Autodesk Inventor part; units mm, degrees
ref_plane "YZ Plane" through (0, 0, 0) normal (1, 0, 0) x (0, 1, 0)
ref_plane "XZ Plane" through (0, 0, 0) normal (0, 1, 0) x (-1, 0, 0)
ref_plane "XY Plane" through (0, 0, 0) normal (0, 0, 1) x (1, 0, 0)
sketch "Sketch1" plane through (0, 0, 0) normal (0, 1, 0) x (-1, 0, 0)
  line L0 (-18.5, 9.5) -> (-18.5, -9.5)
  line L1 (-18.5, -9.5) -> (18.5, -9.5)
  line L2 (18.5, -9.5) -> (18.5, 9.5)
  line L3 (18.5, 9.5) -> (-18.5, 9.5)
  line L4 (-18.5, 9.5) -> (18.5, -9.5) construction
  line L5 (-18.5, -9.5) -> (18.5, 9.5) construction
  point P0 (0, 0)
  dimension "d0" = 19
  dimension "d1" = 37
extrude "Extrusion1" add sketch "Sketch1" along normal blind 1
sketch "Sketch2" plane through (0, 1, 0) normal (0, 1, 0) x (1, 0, 0)
  line L0 (-18.5, 9.5) -> (-18.5, -9.5) construction
  line L1 (18.5, 9.5) -> (-18.5, 9.5) construction
  line L2 (-18.5, -9.5) -> (18.5, 9.5) construction
  line L3 (18.5, -9.5) -> (18.5, 9.5) construction
  line L4 (-18.5, 9.5) -> (18.5, -9.5) construction
  line L5 (-18.5, 0) -> (18.5, 0) construction
  line L6 (0, -9.5) -> (0, 9.5) construction
  line L7 (18.5, 9.5) -> (14.5, 9.5) construction
  line L8 (14.5, 9.5) -> (14.5, 8.5) construction
  line L9 (14.5, 8.5) -> (14.5, 4.5)
  line L10 (14.5, 4.5) -> (4.5, 4.5)
  line L11 (4.5, 4.5) -> (4.5, 8.5)
  line L12 (4.5, 8.5) -> (14.5, 8.5)
  line L13 (4.5, 4.5) -> (14.5, 8.5) construction
  line L14 (4.5, 8.5) -> (14.5, 4.5) construction
  line L15 (6.6893, 4.5) -> (6.6893, 8.5) construction
  line L16 (6.6893, 5.3757) -> (14.5, 5.3757) construction
  line L17 (12.159, 4.5) -> (12.159, 8.5) construction
  line L18 (6.6893, 6.5) -> (12.159, 6.5) construction
  line L19 (6.6893, 8.5) -> (12.159, 8.5)
  line L20 (12.159, 4.5) -> (6.6893, 4.5)
  arc A0 (6.6893, 8.5) -> (6.6893, 4.5) centre (6.6893, 6.5) ccw
  arc A1 (12.159, 4.5) -> (12.159, 8.5) centre (12.159, 6.5) ccw
  line L21 (18.5, 4.5) -> (11.5, 4.5) construction
  line L22 (11.5, 4.5) -> (11.5, 4) construction
  line L23 (11.5, 4) -> (11.5, -2)
  line L24 (11.5, -2) -> (7.5, -2)
  line L25 (7.5, -2) -> (7.5, 4)
  line L26 (7.5, 4) -> (11.5, 4)
  line L27 (7.5, 4) -> (1.5, 4) construction
  line L28 (1.5, 4) -> (-5, 4)
  line L29 (-5, 4) -> (-5, -2.5)
  line L30 (-5, -2.5) -> (1.5, -2.5)
  line L31 (1.5, -2.5) -> (1.5, 4)
  line L32 (-18.5, -9.5) -> (-18.5, -9)
  line L33 (-18.5, -9) -> (-18.5, -8)
  line L34 (-18.5, -8) -> (-18.5, -7.5)
  line L35 (-18.5, -7.5) -> (-18.5, -6.5)
  line L36 (-18.5, -6.5) -> (-18.5, -6)
  line L37 (-18.5, -6) -> (-18.5, -5)
  line L38 (-18.5, -5) -> (-16.5, -5)
  line L39 (-16.5, -5) -> (-16.5, -9)
  line L40 (-16.5, -9) -> (-18.5, -9)
  line L41 (-18.5, -8) -> (-16.5, -8)
  line L42 (-18.5, -7.5) -> (-16.5, -7.5)
  line L43 (-18.5, -6.5) -> (-16.5, -6.5)
  line L44 (-18.5, -6) -> (-16.5, -6)
  point P0 (0, 0)
  point P1 (9.4242, 6.5)
  dimension "d4" = 4
  dimension "d5" = 1
  dimension "d6" = 4
  dimension "d7" = 10
  dimension "d8" = 7
  dimension "d9" = 0.5
  dimension "d10" = 6
  dimension "d11" = 4
  dimension "d12" = 6
  dimension "d13" = 6.5
  dimension "d14" = 6.5
  dimension "d15" = 0.5
  dimension "d16" = 1
  dimension "d17" = 0.5
  dimension "d18" = 1
  dimension "d19" = 0.5
  dimension "d20" = 1
  dimension "d21" = 2
extrude "Extrusion2" add sketch "Sketch2" along normal blind 0.25 contours L9 L10 A1 L12 | A1 L10 A0 L12 | A0 L10 L11 L12 | L23 L24 L25 L26 | L31 L30 L29 L28
extrude "Extrusion3" add sketch "Sketch2" along normal blind 1 contours L33 L41 L39 L40 | L35 L43 L39 L42 | L37 L38 L39 L44
sketch "Sketch3" plane through (-18.5, 0, -9.5) normal (-1, 0, 0) x (0, 0, 1)
  line L0 (19, 0) -> (19, 1)
  line L1 (19, 0) -> (19, 6)
  line L2 (19, 6) -> (13, 6)
  line L3 (13, 6) -> (13, 0)
  line L4 (0, 0) -> (19, 0)
  point P0 (9.5, 0)
  dimension "d26" = 6
  dimension "d27" = 6
extrude "Extrusion4" add sketch "Sketch3" along normal blind 13
sketch "Sketch4" plane through (-31.5, 0, -9.5) normal (-1, 0, 0) x (0, 0, 1)
  line L0 (13, 6) -> (13, 1) construction
  line L1 (19, 0) -> (19, 1) construction
  line L2 (13, 6) -> (19, 0) construction
  line L3 (19, 0) -> (19, 6) construction
  line L4 (19, 6) -> (13, 0) construction
  circle A0 centre (16, 3) radius 2.25
  point P0 (9.5, 0)
  dimension "d30" = 4.5
extrude "Extrusion5" add sketch "Sketch4" along normal blind 1.5
sketch "Sketch5" plane through (-33, 3, 6.5) normal (-1, 0, 0) x (0, 0, 1)
  line L0 (3, -3) -> (3, 3)
  line L1 (3, 3) -> (-3, 3)
  line L2 (-3, 3) -> (-3, -3)
  line L3 (-3, -3) -> (3, -3)
  line L4 (3, -3) -> (-3, 3) construction
  line L5 (3, 3) -> (-3, -3) construction
  point P0 (-6.5, -3)
  point P1 (0, 0)
  dimension "d33" = 6
  dimension "d34" = 6
extrude "Extrusion6" add sketch "Sketch5" along normal blind 6
sketch "Sketch6" plane through (-33, 6, 9.5) normal (0, 1, 0) x (1, 0, 0)
  line L0 (-6, 0) -> (-6, 6) construction
  line L1 (-6, 6) -> (0, 0) construction
  line L2 (0, 0) -> (0, 6) construction
  line L3 (0, 6) -> (-6, 0) construction
  circle A0 centre (-3, 3) radius 3
  point P0 (33, 9.5)
extrude "Extrusion7" add sketch "Sketch6" along normal blind 50
fillet "Fillet1" radius 2 1 edges at (-39, 56, 6.5)
extrude "Extrusion8" add sketch "Sketch2" along normal blind 5 contours A1 L10 A0 L12
fillet "Fillet2" radius 0.5 4 edges at (9.4242, 6, -4.5) (14.159, 6, -6.5) (9.4242, 6, -8.5) (4.6893, 6, -6.5)
properties part number "APC 220"
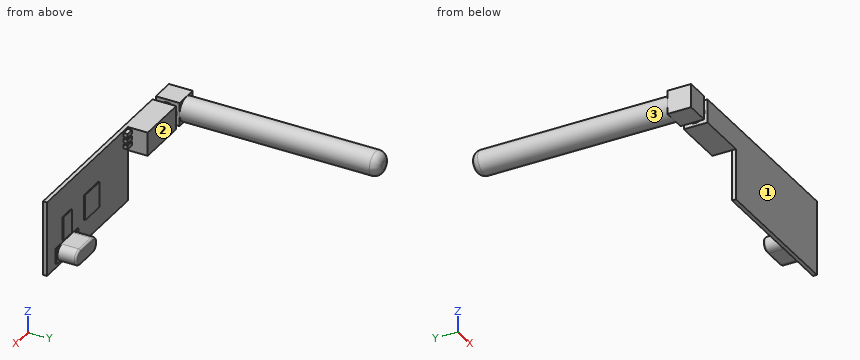
Source: CAD feature listing. Evaluate the final solid. Frame: model axes, mm. Face numbers are marked on the shaded views. A direction names the side the tool comes from. Give positions to 0.01 mm unless a question says otherwise; leave off trailing zeros. Loops run counter-clockwise (first coordinate to the right, second up) from the corner with the lowest first, then second, coordinate; pieces in that order, holes last. Notation, with made-up numbers: (33.5, -19.5) -> (50.5, -19.5) arc R18 ccw to (50.5, 10.5) -> close; hole circle Ø10 at (64.5, 5.25). An arc over 180 degrees is marked (long way). Use a Markdown table: item, result. Add a question column.
(1) Section query B-B (z = -0.75). Output: boundary loops of the cut face in (x, y), then the cut area to 3 significant figures.
(2) Section query D-D (z = -6.5). Output: boundary loops of the cut face in (x, y).
(3) Section query A-A (y = 3). Output: boundary loops of the cut face in (x, z).
(4) Access query for the marked faces 1, 2 and 3. Directions: +Z, -Z, +X, -X, +Y, -Y. A direction counts if a zero-diameter tool reaches every point of the face in a straight line with its end or side. Return the directions, or none.
(5) First-contact query: pin 1 Ø3 at (x, y) = (-37.5, 1.5) entering from -Z; pin 2 Ø4 at (x, z) = (-13.5, 1.5) entering from -Y; pin 3 Ø0.8 at (y, z) = (1.5, 8.5) entering from +X; pin 4 Ø1.2 at (x, z) = (13, -5.5) entering from +Y. Flat tips, straight axial feed; report the tip coordinate or a pass-through.
(6) Ray query, line 1 (Y direction, x = 11.5, z = 3); line 2 (Y direction, x = -29, z = 6.5); line 3 (Z direction, x = -34, y = 51.5). Return the intervals inside material, ascending.
(7) Section query C-C (x = -21). Output: boundary loops of the cut face in (y, z), then the cut area to 3 significant figures.
Checked values:
| question | item | result |
|---|---|---|
| 1 | outline | (-18.5, 0) -> (18.5, 0) -> (18.5, 1) -> (11.5, 1) -> (11.5, 1.25) -> (7.5, 1.25) -> (7.5, 1) -> (1.5, 1) -> (1.5, 1.25) -> (-5, 1.25) -> (-5, 1) -> (-18.5, 1) -> close |
| 1 | area | 39.6 mm^2 |
| 2 | outline | (-18.5, 0) -> (18.5, 0) -> (18.5, 1) -> (14.5, 1) -> (14.5, 1.25) -> (14.16, 1.25) -> (14.16, 5.5) arc R0.5 ccw to (13.66, 6) -> (5.19, 6) arc R0.5 ccw to (4.69, 5.5) -> (4.69, 1.25) -> (4.5, 1.25) -> (4.5, 1) -> (-18.5, 1) -> close |
| 3 | outline | (-39, 3.5) -> (-33, 3.5) -> (-33, 4.25) -> (-31.5, 4.25) -> (-31.5, 3.5) -> (-18.5, 3.5) -> (-18.5, 9.5) -> (-31.5, 9.5) -> (-31.5, 8.75) -> (-33, 8.75) -> (-33, 9.5) -> (-39, 9.5) -> close; (6.69, -8.5) -> (12.16, -8.5) arc R2 ccw to (12.16, -4.5) -> (6.69, -4.5) arc R2 ccw to start |
| 4 | face 1 | +Z, -Z, +X, -X, -Y |
| 4 | face 2 | +Z, -Z, +X, +Y |
| 4 | face 3 | +Y |
| 5 | pin 1 | z = 3.5 |
| 5 | pin 2 | y = 0 |
| 5 | pin 3 | x = -16.5 |
| 5 | pin 4 | y = 6 |
| 6 | line 1 | 0 to 1 |
| 6 | line 2 | 0 to 6 |
| 6 | line 3 | 4.26 to 8.74 |
| 7 | outline | (0, 3.5) -> (6, 3.5) -> (6, 9.5) -> (0, 9.5) -> close |
| 7 | area | 36.0 mm^2 |
